Design review of the part shown in the three views and the two pictorial views. Dimensions are in mm from the part's minimum x, y and z. A direction names the side the tool comes from. Round coordinates to 2 decimals unless told otherwise and drop trailing zeros. Loops run counter-clockwise (first coordinate to the right, second up) from the corner with the lowest first, then second, coordinate; pieces in that order, holes last. Notation, with made-up numbers: (-19, 83) -> (-15, 83) arc R26 cw to (-15, 103) -> close; hole circle Ø6 at (35, 89.25). An arc over 180 degrees is marked (long way). Write each question's results on one line, items separated by ' | '. Start each with the question number.
Item 1: We need section A-A (z = 25.5). Give the boundary of the cut face in (x, y), and give its area (3 significant figures).
Item 2: Tool access review of the marked faces 1 and 2: name each direction out of +Z, -Z, +X, -X, +Y, -Y from which nothing blocks a thin tool from reaching the whole face with its end or side.
Item 3: We need section D-D (z = 34). Give the boundary of the cut face in (x, y), and give its area (3 significant figures).
Item 4: We need section B-B (x = 23.5). Give the boundary of the cut face in (y, z), and give its area (4 significant figures).
Item 5: For L1, parallel to Z at x = 30, y = 33.5; L2, parallel to Z at x = 30, y = 28; L3, parallel to Y at x = 26, z = 37.5, list the stretches that pass through material, from the lowest coordinate up. Write a range as from..to.
Item 6: Clearance check with flat-ended pins moving along their axes: pin 1 Ø2.5 at (x, z) = (29.5, 24.5) entering from -Y; pin 2 Ø19 at (x, z) = (26, 34) entering from -Y; pin 3 Ø4 at (x, y) = (29.5, 22.5) entering from +Z. State where each tip first meets the part, or that it passes through.
Item 7: We need section C-C (y = 11.5). Give the boundary of the cut face in (x, z).
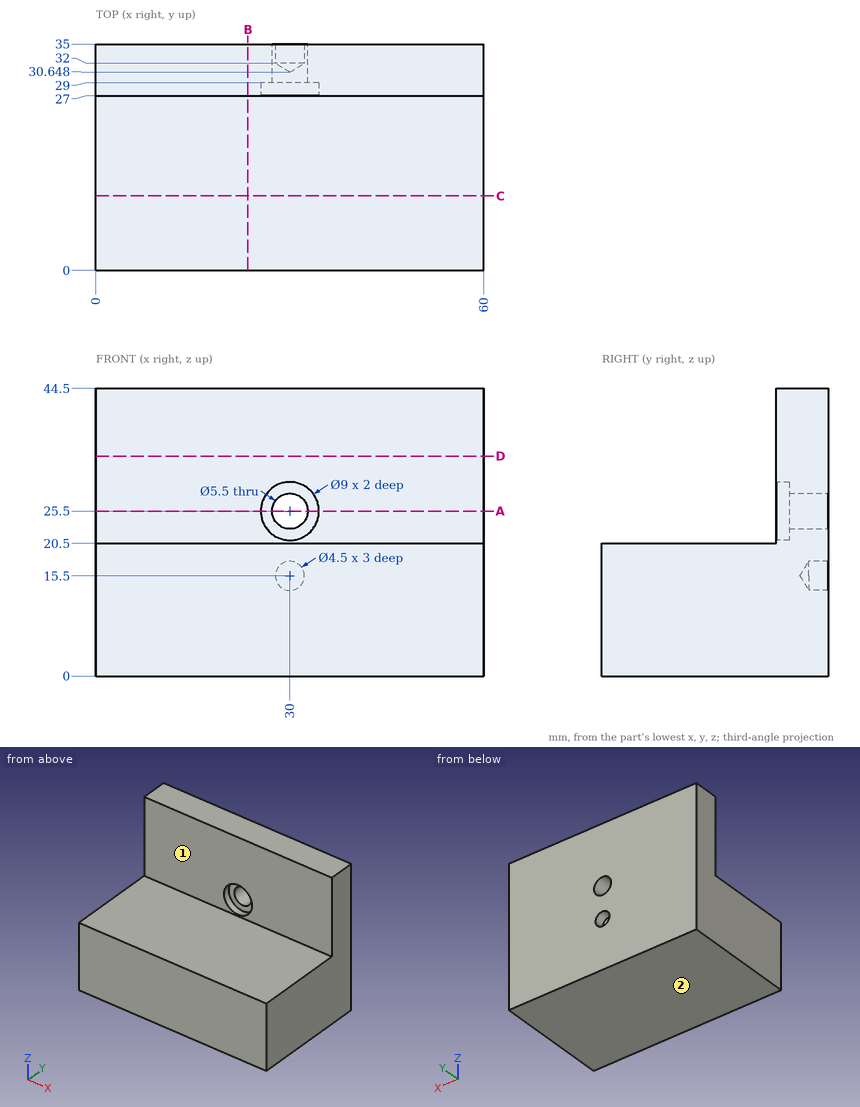
Here are the results:
1) outline: (0, 27) -> (25.5, 27) -> (25.5, 29) -> (27.25, 29) -> (27.25, 35) -> (0, 35) -> close; (32.75, 29) -> (34.5, 29) -> (34.5, 27) -> (60, 27) -> (60, 35) -> (32.75, 35) -> close | area: 429 mm2
2) face 1: +Z, +X, -X, -Y | face 2: -Z, +X, -X, +Y, -Y
3) outline: (0, 27) -> (60, 27) -> (60, 35) -> (0, 35) -> close | area: 480 mm2
4) outline: (0, 0) -> (35, 0) -> (35, 44.5) -> (27, 44.5) -> (27, 20.5) -> (0, 20.5) -> close | area: 909.5 mm2
5) L1: z = 0..13.25, 17.75..22.75, 28.25..44.5 | L2: z = 0..21, 30..44.5 | L3: y = 27..35
6) pin 1: passes through | pin 2: stops at y = 27 | pin 3: stops at z = 20.5
7) outline: (0, 0) -> (60, 0) -> (60, 20.5) -> (0, 20.5) -> close
